For this review, take the finished solid that the model builds, in its own axes (mm). A direction names the side the tool comes from. Give positions to 0.01 mm unless a question says otherwise; leave off trailing zeros. Write each loop counter-clockwise with the first axis right and the second up, starting at its lowest first coordinate (ties: lowest second). Pieces come first, ordered by that corner, then holes. Notation, with made-up numbers: (-15.75, 57.5) -> (28.25, 57.5) arc R23 ccw to (28.25, 85.5) -> close; hole circle Ø9 at (24.25, -26.75). An arc over 180 degrees is marked (long way). Answer as CSV lines item,"result".
```python
from build123d import *

# Parameters (mm, degrees)
F0_R     = 13.579833
F1_DEPTH = 57.404
F2_T     = -2.54
F4_R     = 11.66888
F5_DEPTH = 44.45
F6_R     = 11.401717
F7_DEPTH = 42.672


with BuildPart() as f1:
    # F0 (on Front) → F1 (new body, symmetric)
    with BuildSketch(Plane.XZ):
        Circle(F0_R)
    extrude(amount=F1_DEPTH, both=True)

    # F2
    f2_openings = [f1.faces().sort_by_distance(p)[0] for p in [
        (0, -57.404, 0),
        (0, 57.404, 0),
    ]]
    offset(amount=F2_T, openings=f2_openings)

    # F4 (on offset) → F5 (join)
    with BuildSketch(Plane.XY.offset(7.874)):
        Circle(F4_R)
    extrude(amount=F5_DEPTH)

    # F6 (on face) → F7 (cut)
    with BuildSketch(Plane.XY.offset(52.324)):
        Circle(F6_R)
    extrude(amount=-F7_DEPTH, mode=Mode.SUBTRACT)


solid = f1.part
```
Q1. Add section D-D (z = 24.5). Write out the cut boundary in (x, y).
Answer block:
outline,"circle Ø23.34 at (0, 0); hole circle Ø22.8 at (0, 0)"
Q2. Add section C-C (x = 0). Write out the cut boundary in (y, z).
Answer block:
outline,"(-57.4, -13.58) -> (57.4, -13.58) -> (57.4, -11.04) -> (-57.4, -11.04) -> close; (-57.4, 11.04) -> (-11.67, 11.04) -> (-11.67, 7.87) -> (11.67, 7.87) -> (11.67, 11.04) -> (57.4, 11.04) -> (57.4, 13.58) -> (11.67, 13.58) -> (11.67, 52.32) -> (11.4, 52.32) -> (11.4, 9.65) -> (-11.4, 9.65) -> (-11.4, 52.32) -> (-11.67, 52.32) -> (-11.67, 13.58) -> (-57.4, 13.58) -> close"
Q3. To check wall thickness, follow probe 1 along Y at (x, z) = (0, 38); probe 2 along X at (y, z) = (-2, -0.5); probe 3 along Z at (x, y) = (-5, -47). State the ranges of each line that lie inside material, in increasing order. Write a range as [from, to].
Answer block:
probe 1,"y = [-11.67, -11.4], [11.4, 11.67]"
probe 2,"x = [-13.57, -11.03], [11.03, 13.57]"
probe 3,"z = [-12.63, -9.84], [9.84, 12.63]"
Q4. Add section A-A (z = 0). Write out the cut boundary in (x, y), plus the area to 3 significant figures.
Answer block:
outline,"(-13.58, -57.4) -> (-11.04, -57.4) -> (-11.04, 57.4) -> (-13.58, 57.4) -> close; (11.04, -57.4) -> (13.58, -57.4) -> (13.58, 57.4) -> (11.04, 57.4) -> close"
area,"583 mm2"
Q5. For faces 1 (the cylindrical face through (-2.53, -11.39, 29.79)), 2 (the flat face through (-2.1, -57.404, 11.1)), 3 (the cylindrical face through (-2.944, -0.804, -13.257)), 4 (the flat face through (0, 0, 7.874)), list the 3-axis set-ups (+Z, -Z, +X, -X, +Y, -Y) from which the entire face can be reached by the end or side of a thin tool; tool diameter is ignored.
Answer block:
face 1,"+Z"
face 2,"+Z, -Z, +X, -X, -Y"
face 3,"none"
face 4,"+Y, -Y"
Q6. Draft analysis for pull direction Z (two halves, no side actions). For faces 5 (the cylindrical face through (-2.39, -0.8, -10.78)), 6 (the flat face through (-2.1, 57.404, 11.1)), 7 (the flat face through (0, 0, 9.652)), state which applies: released by +Z, released by -Z, zero draft, split by the parting line, or undercut.
Answer block:
face 5,"undercut"
face 6,"zero draft"
face 7,"released by +Z"
Q7. Add section B-B (y = 0). Write out the cut boundary in (x, z), plus the area to 3 significant figures.
Answer block:
outline,"(-11.67, 7.87) -> (-11.06, 7.87) arc R13.58 ccw (long way) to (11.06, 7.87) -> (11.67, 7.87) -> (11.67, 52.32) -> (11.4, 52.32) -> (11.4, 9.65) -> (-11.4, 9.65) -> (-11.4, 52.32) -> (-11.67, 52.32) -> close; hole (-7.74, 7.87) arc R11.04 ccw (long way) to (7.74, 7.87) -> close"
area,"206 mm2"
Q8. Clearance check with flat-ended pins moving along their axes: pin 1 (1 mm diameter, centred on y = -13.5, z = 8, fed in from -X); pin 2 (1.5 mm diameter, centred on y = -7.5, z = 28.5, fed in from +X); pin 3 (5 mm diameter, centred on x = 0.5, z = 23, fed in from +Y). State where each tip first meets the part, or that it passes through.
Answer block:
pin 1,"stops at x = -11.32"
pin 2,"stops at x = 9.52"
pin 3,"stops at y = 11.67"
